Input: part model. Units: mm. Frame: model coordinates. A direction names the side the tool comes from. Give positions to 0.01 mm unless a question says otherwise; leave off trailing zeros. Loops run counter-clockwise (first coordinate to the right, second up) from the corner with the lowest first, then second, coordinate; pieces in that order, holes last. Notation, with made-up numbers: M 28.25,54 L 78.25,54 A15 cw 78.25,79 Z; hole C -7.75,11.25 d2. An arc over 180 degrees is marked long. Answer as a JSON object with one key per item and string values. Group by question number.
1) Draft query along X for faces 1 (the cylindrical face through (19.745, 3.185, 1.972)), 2 (the flat face through (-27, 0, 0)), 3 (the cylindrical face through (-0.07, -26.25, 1.97)). Return one class per face: +X half, -X half, draft (parallel to the pull), parting line (faces both ways), or undercut.
2) First-contact query: P1, Ø0.8, axis at x = 17, z = -0.5, coming from the -Y side; P2, Ø2, axis at x = -3.5, y = 13, coming from the +Z side; P3, Ø1.5, axis at x = -15, z = 0.5, coming from the +Y side; P4, Ø3, axis at x = -7.5, y = 19.5, coming from the +Z side. Flat tips, straight axial feed; report the tip coordinate or a pass-through.
3) Section query A-A on x = 0. Return loops of the section in (y, z).
4) Section query D-D on y = 22. Return loops of the section in (x, z), plus the area to 3 significant figures.
5) Access query for faces 4 (the flat face through (-4, 7.5, 2)), 5 (the flat face through (-7.5, -4, 2)), 6 (the cylindrical face through (3.125, 19.754, 1.972)), 7 (the flat face through (4, 7.5, 2)), 8 (the flat face through (-5.273, 20, 1)). Directions: +Z, -Z, +X, -X, +Y, -Y. A direction counts if a zero-diameter tool reaches every point of the face in a straight line with its end or side. Return the directions, or none.
6) Ray query, L1, parallel to Y at x = 2, z = 2.7; L2, parallel to Z at x = 17.5, y = 2.5; L3, parallel to Y at x = -10.5, z = 3.7. Return the intervals inside material, ascending.
7) Section query B-B on x = 10. Return loops of the section in (y, z), plus the area to 3 significant figures.
from build123d import *

# Parameters (mm, degrees)
F0_R     = 4.1
F0_W     = 2.2272727273
F0_H     = 2.2272727273
F1_DEPTH = 1
F2_DEPTH = 4


with BuildPart() as f1:
    # F0 (on Top) → F1 (new body)
    with BuildSketch(Plane.XY):
        with BuildLine():
            Line((5.2727272727, 19.292442746), (5.2727272727, 25.7149926523))
            ThreePointArc((5.2727272727, 25.7149926523), (0, 26.25), (-5.2727272727, 25.7149926523))
            Line((-5.2727272727, 25.7149926523), (-5.2727272727, 19.292442746))
            ThreePointArc((-5.2727272727, 19.292442746), (-3.1548760073, 19.7496014486), (-1, 19.9749843554))
            ThreePointArc((-1, 19.9749843554), (0, 20), (1, 19.9749843554))
            ThreePointArc((1, 19.9749843554), (3.1548760073, 19.7496014486), (5.2727272727, 19.292442746))
        make_face()
        with BuildLine():
            ThreePointArc((-25.7149926523, -5.2727272727), (-26.25, 0), (-25.7149926523, 5.2727272727))
            Line((-25.7149926523, 5.2727272727), (-28.516632815, 5.2727272727))
            ThreePointArc((-28.516632815, 5.2727272727), (-29, 0), (-28.516632815, -5.2727272727))
            Line((-28.516632815, -5.2727272727), (-25.7149926523, -5.2727272727))
        make_face()
        with BuildLine():
            ThreePointArc((-5.2727272727, 25.7149926523), (0, 26.25), (5.2727272727, 25.7149926523))
            Line((5.2727272727, 25.7149926523), (5.2727272727, 28.516632815))
            ThreePointArc((5.2727272727, 28.516632815), (0, 29), (-5.2727272727, 28.516632815))
            Line((-5.2727272727, 28.516632815), (-5.2727272727, 25.7149926523))
        make_face()
        with BuildLine():
            ThreePointArc((25.7149926523, 5.2727272727), (26.1159056623, 2.6499002696), (26.25, 0))
            ThreePointArc((26.25, 0), (26.1159056623, -2.6499002696), (25.7149926523, -5.2727272727))
            Line((25.7149926523, -5.2727272727), (28.516632815, -5.2727272727))
            ThreePointArc((28.516632815, -5.2727272727), (28.8789053778, -2.6474183995), (29, 0))
            ThreePointArc((29, 0), (28.8789053778, 2.6474183995), (28.516632815, 5.2727272727))
            Line((28.516632815, 5.2727272727), (25.7149926523, 5.2727272727))
        make_face()
        with BuildLine():
            Line((5.2727272727, -28.516632815), (5.2727272727, -25.7149926523))
            ThreePointArc((5.2727272727, -25.7149926523), (0, -26.25), (-5.2727272727, -25.7149926523))
            Line((-5.2727272727, -25.7149926523), (-5.2727272727, -28.516632815))
            ThreePointArc((-5.2727272727, -28.516632815), (0, -29), (5.2727272727, -28.516632815))
        make_face()
        with BuildLine():
            Line((-7.5, 5.2727272727), (-19.292442746, 5.2727272727))
            ThreePointArc((-19.292442746, 5.2727272727), (-19.7496014486, 3.1548760073), (-19.9749843554, 1))
            Line((-19.9749843554, 1), (-7.5, 1))
            Line((-7.5, 1), (-7.5, 5.2727272727))
        make_face()
        Polygon((7.5, 1), (7.5, 5.2727272727), (5.2727272727, 5.2727272727), (5.2727272727, 7.5), (1, 7.5), (-1, 7.5), (-5.2727272727, 7.5), (-5.2727272727, 5.2727272727), (-7.5, 5.2727272727), (-7.5, 1), (-7.5, -1), (-7.5, -5.2727272727), (-5.2727272727, -5.2727272727), (-5.2727272727, -7.5), (-1, -7.5), (1, -7.5), (5.2727272727, -7.5), (5.2727272727, -5.2727272727), (7.5, -5.2727272727), (7.5, -1), align=None)
        Circle(F0_R, mode=Mode.SUBTRACT)
        with BuildLine():
            ThreePointArc((-1, 19.9749843554), (-3.1548760073, 19.7496014486), (-5.2727272727, 19.292442746))
            Line((-5.2727272727, 19.292442746), (-5.2727272727, 7.5))
            Line((-5.2727272727, 7.5), (-1, 7.5))
            Line((-1, 7.5), (-1, 19.9749843554))
        make_face()
        with BuildLine():
            ThreePointArc((19.9749843554, 1), (19.7496014486, 3.1548760073), (19.292442746, 5.2727272727))
            Line((19.292442746, 5.2727272727), (7.5, 5.2727272727))
            Line((7.5, 5.2727272727), (7.5, 1))
            Line((7.5, 1), (19.9749843554, 1))
        make_face()
        with BuildLine():
            ThreePointArc((25.7149926523, -5.2727272727), (26.1159056623, -2.6499002696), (26.25, 0))
            ThreePointArc((26.25, 0), (26.1159056623, 2.6499002696), (25.7149926523, 5.2727272727))
            Line((25.7149926523, 5.2727272727), (19.292442746, 5.2727272727))
            ThreePointArc((19.292442746, 5.2727272727), (19.7496014486, 3.1548760073), (19.9749843554, 1))
            ThreePointArc((19.9749843554, 1), (19.9937451108, 0.5001564212), (20, 0))
            ThreePointArc((20, 0), (19.9937451108, -0.5001564212), (19.9749843554, -1))
            ThreePointArc((19.9749843554, -1), (19.7496014486, -3.1548760073), (19.292442746, -5.2727272727))
            Line((19.292442746, -5.2727272727), (25.7149926523, -5.2727272727))
        make_face()
        with BuildLine():
            Line((-5.2727272727, -7.5), (-5.2727272727, -19.292442746))
            ThreePointArc((-5.2727272727, -19.292442746), (-3.1548760073, -19.7496014486), (-1, -19.9749843554))
            Line((-1, -19.9749843554), (-1, -7.5))
            Line((-1, -7.5), (-5.2727272727, -7.5))
        make_face()
        with BuildLine():
            ThreePointArc((-5.2727272727, -25.7149926523), (0, -26.25), (5.2727272727, -25.7149926523))
            Line((5.2727272727, -25.7149926523), (5.2727272727, -19.292442746))
            ThreePointArc((5.2727272727, -19.292442746), (3.1548760073, -19.7496014486), (1, -19.9749843554))
            ThreePointArc((1, -19.9749843554), (0, -20), (-1, -19.9749843554))
            ThreePointArc((-1, -19.9749843554), (-3.1548760073, -19.7496014486), (-5.2727272727, -19.292442746))
            Line((-5.2727272727, -19.292442746), (-5.2727272727, -25.7149926523))
        make_face()
        with BuildLine():
            Line((-19.292442746, 5.2727272727), (-25.7149926523, 5.2727272727))
            ThreePointArc((-25.7149926523, 5.2727272727), (-26.25, 0), (-25.7149926523, -5.2727272727))
            Line((-25.7149926523, -5.2727272727), (-19.292442746, -5.2727272727))
            ThreePointArc((-19.292442746, -5.2727272727), (-19.7496014486, -3.1548760073), (-19.9749843554, -1))
            ThreePointArc((-19.9749843554, -1), (-20, 0), (-19.9749843554, 1))
            ThreePointArc((-19.9749843554, 1), (-19.7496014486, 3.1548760073), (-19.292442746, 5.2727272727))
        make_face()
        with Locations((-6.3863636364, 6.3863636364)):
            Rectangle(F0_W, F0_H)
        with Locations((-6.3863636364, -6.3863636364)):
            Rectangle(F0_W, F0_H)
        with Locations((6.3863636364, -6.3863636364)):
            Rectangle(F0_W, F0_H)
        with Locations((6.3863636364, 6.3863636364)):
            Rectangle(F0_W, F0_H)
        with BuildLine():
            ThreePointArc((20, 0), (19.9937451108, 0.5001564212), (19.9749843554, 1))
            Line((19.9749843554, 1), (7.5, 1))
            Line((7.5, 1), (7.5, -1))
            Line((7.5, -1), (19.9749843554, -1))
            ThreePointArc((19.9749843554, -1), (19.9937451108, -0.5001564212), (20, 0))
        make_face()
        with BuildLine():
            Line((7.5, -5.2727272727), (19.292442746, -5.2727272727))
            ThreePointArc((19.292442746, -5.2727272727), (19.7496014486, -3.1548760073), (19.9749843554, -1))
            Line((19.9749843554, -1), (7.5, -1))
            Line((7.5, -1), (7.5, -5.2727272727))
        make_face()
        with BuildLine():
            ThreePointArc((-19.9749843554, -1), (-19.7496014486, -3.1548760073), (-19.292442746, -5.2727272727))
            Line((-19.292442746, -5.2727272727), (-7.5, -5.2727272727))
            Line((-7.5, -5.2727272727), (-7.5, -1))
            Line((-7.5, -1), (-19.9749843554, -1))
        make_face()
        with BuildLine():
            Line((-7.5, 1), (-19.9749843554, 1))
            ThreePointArc((-19.9749843554, 1), (-20, 0), (-19.9749843554, -1))
            Line((-19.9749843554, -1), (-7.5, -1))
            Line((-7.5, -1), (-7.5, 1))
        make_face()
        with BuildLine():
            Line((1, 7.5), (1, 19.9749843554))
            ThreePointArc((1, 19.9749843554), (0, 20), (-1, 19.9749843554))
            Line((-1, 19.9749843554), (-1, 7.5))
            Line((-1, 7.5), (1, 7.5))
        make_face()
        with BuildLine():
            Line((5.2727272727, 7.5), (5.2727272727, 19.292442746))
            ThreePointArc((5.2727272727, 19.292442746), (3.1548760073, 19.7496014486), (1, 19.9749843554))
            Line((1, 19.9749843554), (1, 7.5))
            Line((1, 7.5), (5.2727272727, 7.5))
        make_face()
        with BuildLine():
            ThreePointArc((1, -19.9749843554), (3.1548760073, -19.7496014486), (5.2727272727, -19.292442746))
            Line((5.2727272727, -19.292442746), (5.2727272727, -7.5))
            Line((5.2727272727, -7.5), (1, -7.5))
            Line((1, -7.5), (1, -19.9749843554))
        make_face()
        with BuildLine():
            ThreePointArc((-1, -19.9749843554), (0, -20), (1, -19.9749843554))
            Line((1, -19.9749843554), (1, -7.5))
            Line((1, -7.5), (-1, -7.5))
            Line((-1, -7.5), (-1, -19.9749843554))
        make_face()
    extrude(amount=-F1_DEPTH)

    # F0 (on Top) → F2 (join)
    with BuildSketch(Plane.XY):
        with BuildLine():
            ThreePointArc((25.7149926523, -5.2727272727), (26.1159056623, -2.6499002696), (26.25, 0))
            ThreePointArc((26.25, 0), (26.1159056623, 2.6499002696), (25.7149926523, 5.2727272727))
            Line((25.7149926523, 5.2727272727), (19.292442746, 5.2727272727))
            ThreePointArc((19.292442746, 5.2727272727), (19.7496014486, 3.1548760073), (19.9749843554, 1))
            ThreePointArc((19.9749843554, 1), (19.9937451108, 0.5001564212), (20, 0))
            ThreePointArc((20, 0), (19.9937451108, -0.5001564212), (19.9749843554, -1))
            ThreePointArc((19.9749843554, -1), (19.7496014486, -3.1548760073), (19.292442746, -5.2727272727))
            Line((19.292442746, -5.2727272727), (25.7149926523, -5.2727272727))
        make_face()
        with BuildLine():
            Line((5.2727272727, 19.292442746), (5.2727272727, 25.7149926523))
            ThreePointArc((5.2727272727, 25.7149926523), (0, 26.25), (-5.2727272727, 25.7149926523))
            Line((-5.2727272727, 25.7149926523), (-5.2727272727, 19.292442746))
            ThreePointArc((-5.2727272727, 19.292442746), (-3.1548760073, 19.7496014486), (-1, 19.9749843554))
            ThreePointArc((-1, 19.9749843554), (0, 20), (1, 19.9749843554))
            ThreePointArc((1, 19.9749843554), (3.1548760073, 19.7496014486), (5.2727272727, 19.292442746))
        make_face()
        with BuildLine():
            Line((-19.292442746, 5.2727272727), (-25.7149926523, 5.2727272727))
            ThreePointArc((-25.7149926523, 5.2727272727), (-26.25, 0), (-25.7149926523, -5.2727272727))
            Line((-25.7149926523, -5.2727272727), (-19.292442746, -5.2727272727))
            ThreePointArc((-19.292442746, -5.2727272727), (-19.7496014486, -3.1548760073), (-19.9749843554, -1))
            ThreePointArc((-19.9749843554, -1), (-20, 0), (-19.9749843554, 1))
            ThreePointArc((-19.9749843554, 1), (-19.7496014486, 3.1548760073), (-19.292442746, 5.2727272727))
        make_face()
        with BuildLine():
            ThreePointArc((-5.2727272727, -25.7149926523), (0, -26.25), (5.2727272727, -25.7149926523))
            Line((5.2727272727, -25.7149926523), (5.2727272727, -19.292442746))
            ThreePointArc((5.2727272727, -19.292442746), (3.1548760073, -19.7496014486), (1, -19.9749843554))
            ThreePointArc((1, -19.9749843554), (0, -20), (-1, -19.9749843554))
            ThreePointArc((-1, -19.9749843554), (-3.1548760073, -19.7496014486), (-5.2727272727, -19.292442746))
            Line((-5.2727272727, -19.292442746), (-5.2727272727, -25.7149926523))
        make_face()
        with BuildLine():
            Line((1, 7.5), (1, 19.9749843554))
            ThreePointArc((1, 19.9749843554), (0, 20), (-1, 19.9749843554))
            Line((-1, 19.9749843554), (-1, 7.5))
            Line((-1, 7.5), (1, 7.5))
        make_face()
        with BuildLine():
            Line((-7.5, 1), (-19.9749843554, 1))
            ThreePointArc((-19.9749843554, 1), (-20, 0), (-19.9749843554, -1))
            Line((-19.9749843554, -1), (-7.5, -1))
            Line((-7.5, -1), (-7.5, 1))
        make_face()
        with BuildLine():
            ThreePointArc((20, 0), (19.9937451108, 0.5001564212), (19.9749843554, 1))
            Line((19.9749843554, 1), (7.5, 1))
            Line((7.5, 1), (7.5, -1))
            Line((7.5, -1), (19.9749843554, -1))
            ThreePointArc((19.9749843554, -1), (19.9937451108, -0.5001564212), (20, 0))
        make_face()
        with BuildLine():
            ThreePointArc((-1, -19.9749843554), (0, -20), (1, -19.9749843554))
            Line((1, -19.9749843554), (1, -7.5))
            Line((1, -7.5), (-1, -7.5))
            Line((-1, -7.5), (-1, -19.9749843554))
        make_face()
        Polygon((7.5, 1), (7.5, 5.2727272727), (5.2727272727, 5.2727272727), (5.2727272727, 7.5), (1, 7.5), (-1, 7.5), (-5.2727272727, 7.5), (-5.2727272727, 5.2727272727), (-7.5, 5.2727272727), (-7.5, 1), (-7.5, -1), (-7.5, -5.2727272727), (-5.2727272727, -5.2727272727), (-5.2727272727, -7.5), (-1, -7.5), (1, -7.5), (5.2727272727, -7.5), (5.2727272727, -5.2727272727), (7.5, -5.2727272727), (7.5, -1), align=None)
        Circle(F0_R, mode=Mode.SUBTRACT)
        with Locations((-6.3863636364, 6.3863636364)):
            Rectangle(F0_W, F0_H)
        with Locations((-6.3863636364, -6.3863636364)):
            Rectangle(F0_W, F0_H)
        with Locations((6.3863636364, -6.3863636364)):
            Rectangle(F0_W, F0_H)
        with Locations((6.3863636364, 6.3863636364)):
            Rectangle(F0_W, F0_H)
    extrude(amount=F2_DEPTH)


solid = f1.part
Output:
{
 "1": {"face 1": "undercut", "face 2": "draft", "face 3": "parting line"},
 "2": {"P1": "stops at y = -5.27", "P2": "stops at z = 0", "P3": "stops at y = 5.27", "P4": "passes through"},
 "3": {"outline": "M -29,-1 L -4.1,-1 L -4.1,4 L -26.25,4 L -26.25,0 L -29,0 Z; M 4.1,-1 L 29,-1 L 29,0 L 26.25,0 L 26.25,4 L 4.1,4 Z"},
 "4": {"outline": "M -5.27,-1 L 5.27,-1 L 5.27,4 L -5.27,4 Z", "area": "52.7 mm^2"},
 "5": {"face 4": "+Z, -X", "face 5": "+Z, -Y", "face 6": "+Z", "face 7": "+Z, +X", "face 8": "+Z, -Z, -X, +Y"},
 "6": {"L1": "y = -26.17 to -19.9, -7.5 to -3.58, 3.58 to 7.5, 19.9 to 26.17", "L2": "z = -1 to 0", "L3": "y = -1 to 1"},
 "7": {"outline": "M -5.27,-1 L 5.27,-1 L 5.27,0 L 1,0 L 1,4 L -1,4 L -1,0 L -5.27,0 Z", "area": "18.5 mm^2"}
}
